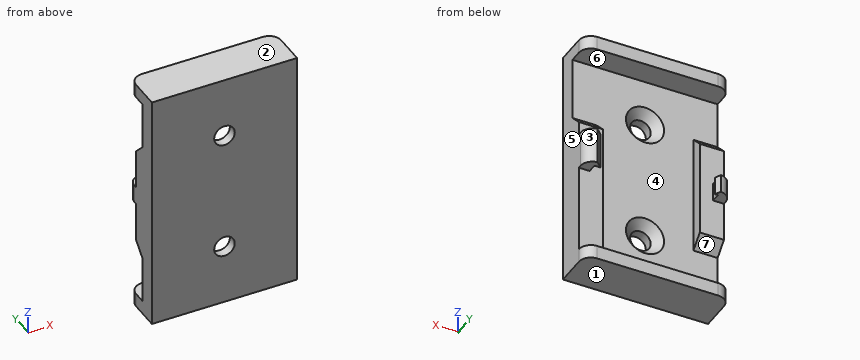
Autodesk Inventor part; units mm, degrees
ref_plane "YZ Plane" through (0, 0, 0) normal (1, 0, 0) x (0, 1, 0)
ref_plane "XZ Plane" through (0, 0, 0) normal (0, 1, 0) x (-1, 0, 0)
ref_plane "XY Plane" through (0, 0, 0) normal (0, 0, 1) x (1, 0, 0)
sketch "Skizze1" plane through (0, 0, 0) normal (0, 1, 0) x (-1, 0, 0)
  line L0 (0, 0) -> (24, 0)
  line L1 (24, 0) -> (24, -40)
  line L2 (24, -40) -> (0, -40)
  line L3 (0, -40) -> (0, 0)
  dimension "d0" = 40
  dimension "d1" = 24
extrude "Extrusion1" add sketch "Skizze1" along normal blind 3
sketch "Skizze2" plane through (0, 3, 0) normal (0, 1, 0) x (1, 0, 0)
  line L0 (-24, 40) -> (-24, 0)
  line L1 (0, 0) -> (0, 40)
  line L2 (-24, 0) -> (0, 0)
  line L3 (0, 0) -> (0, 2.25)
  line L4 (0, 2.25) -> (-24, 2.25)
  line L5 (-24, 2.25) -> (-24, 0)
  line L6 (0, 40) -> (-24, 40)
  line L7 (-24, 40) -> (0, 40)
  line L8 (0, 40) -> (0, 37.75)
  line L9 (0, 37.75) -> (-24, 37.75)
  line L10 (-24, 37.75) -> (-24, 40)
  dimension "d4" = 2.25
  dimension "d5" = 2.25
extrude "Extrusion2" add sketch "Skizze2" along normal blind 4 contours L6 L1 L9 L0 | L4 L1 L2 L0
sketch "Skizze4" plane through (0, 3, 0) normal (0, 1, 0) x (1, 0, 0)
  line L0 (0, 2.25) -> (-24, 2.25)
  line L1 (0, 2.25) -> (-1.8184, 2.25)
  line L2 (0, 37.75) -> (-1.8184, 37.75)
  line L3 (-24.0183, 2.25) -> (-21.7244, 2.25)
  line L4 (-24, 37.75) -> (-21.1801, 37.75)
  line L5 (0, 37.75) -> (-4, 37.75)
  line L6 (-4, 37.75) -> (-4, 12.75)
  line L7 (-4, 12.75) -> (0, 12.75)
  line L8 (0, 12.75) -> (0, 37.75)
  line L9 (-24, 37.75) -> (-24, 2.25)
  line L10 (-24, 10) -> (-20, 10)
  line L11 (-20, 10) -> (-20, 30)
  line L12 (-20, 30) -> (-24, 30)
  line L13 (-24, 30) -> (-24, 10)
  line L14 (-24, 0) -> (0, 0)
  dimension "d25" = 25
  dimension "d26" = 4
  dimension "d27" = 4
  dimension "d29" = 20
  dimension "d30" = 10
extrude "Extrusion4" add sketch "Skizze4" along normal blind 2
sketch "Skizze5" plane through (0, 5, 0) normal (0, 1, 0) x (1, 0, 0)
  line L0 (-24, 30) -> (-24, 10)
  line L1 (-24, 20) -> (0, 20)
  line L2 (0, 0) -> (0, 40)
  line L3 (-24, 18.5) -> (-22.2, 18.5)
  line L4 (-22.2, 18.5) -> (-22.2, 21.5)
  line L5 (-22.2, 21.5) -> (-24, 21.5)
  line L6 (-24, 21.5) -> (-24, 18.5)
  line L7 (0, 17) -> (-1.8, 17)
  line L8 (-1.8, 17) -> (-1.8, 23)
  line L9 (-1.8, 23) -> (0, 23)
  line L10 (0, 23) -> (0, 17)
  point P0 (-23.1, 18.5)
  point P1 (0, 23)
  dimension "d33" = 3
  dimension "d34" = 1.8
  dimension "d35" = 1.8
  dimension "d36" = 6
extrude "Extrusion5" add sketch "Skizze5" along normal blind 2.5
sketch "Skizze6" plane through (-1.8, 5, -23) normal (-1, 0, 0) x (0, 0, 1)
  line L0 (0, 0) -> (0, 2.5)
  line L1 (6, 0) -> (6, 2.5)
  line L2 (0, 2.5) -> (6, 2.5)
  line L3 (6, 2.5) -> (6, 1.5)
  line L4 (6, 1.5) -> (0, 1.5)
  line L5 (0, 1.5) -> (0, 2.5)
  point P0 (23, -5)
  point P1 (0, 1.5)
  dimension "d39" = 1
extrude "Extrusion6" add sketch "Skizze6" along normal blind 1
sketch "Skizze7" plane through (0, 5, -23) normal (0, 0, -1) x (-1, 0, 0)
  line L0 (2.8, 2.5) -> (2.8, 1.5)
  line L1 (2.8, 1.5) -> (1.8, 2.5)
  line L2 (0, 2.5) -> (2.8, 2.5)
  line L3 (1.8, 2.5) -> (2.8, 2.5)
  line L4 (2.8, 2.5) -> (2.8, 1.5)
  point P0 (0, -5)
  dimension "d42" = 1
  dimension "d43" = 1
extrude "Extrusion7" cut sketch "Skizze7" against normal blind 10
sketch "Skizze9" plane through (-22.2, 5, -18.5) normal (1, 0, 0) x (0, 0, -1)
  line L0 (0, 0) -> (0, 2.5)
  line L1 (3, 0) -> (3, 2.5)
  line L2 (0, 2.5) -> (3, 2.5)
  line L3 (3, 2.5) -> (3, 1.5)
  line L4 (3, 1.5) -> (0, 1.5)
  line L5 (0, 1.5) -> (0, 2.5)
  line L6 (3, 0) -> (0, 0)
  point P0 (-18.5, -5)
  point P1 (0, 1.5)
  dimension "d46" = 1.5
extrude "Extrusion8" add sketch "Skizze9" along normal blind 0.5 contours L0 L2 L1 L4
sketch "Skizze11" plane through (-22.2, 5, -21.5) normal (0, 0, -1) x (-1, 0, 0)
  line L0 (-0.5, 2.5) -> (-0.5, 1.5)
  line L1 (-0.5, 1.5) -> (0, 2.5)
  line L2 (1.8, 2.5) -> (-0.5, 2.5)
  line L3 (-0.5, 1.5) -> (-0.5, 2.5)
  line L4 (-0.5, 2.5) -> (0, 2.5)
  point P0 (-22.2, -5)
  dimension "d49" = 0.5
extrude "Extrusion9" cut sketch "Skizze11" against normal blind 10
chamfer "Fasen1" distance 2 angle 45 3 edges at (-22, 5, -30) (-22, 5, -10) (-2, 5, -12.75)
fillet "Rundung1" radius 2 6 edges at (0, 7.5, -20) (-24, 7.5, -20) (-24, 7, -1.125) (0, 7, -1.125) (-24, 7, -38.875) (0, 7, -38.875)
sketch "Skizze12" plane through (0, 3, 0) normal (0, 1, 0) x (1, 0, 0)
  line L0 (-24, 0) -> (0, 0)
  line L1 (-12, 0) -> (-12, 40)
  line L2 (0, 40) -> (-24, 40)
  circle A0 centre (-12, 10) radius 2
  circle A1 centre (-12, 30) radius 2
  line L3 (-24, 40) -> (-24, 0)
  line L4 (-24, 20) -> (0, 20) construction
  line L5 (0, 17) -> (0, 23)
  dimension "d56" = 4
  dimension "d57" = 4
  dimension "d58" = 20
hole "Bohrung1" at (-12, 3, -10) at (-12, 3, -30) direction (0, -1, 0) diameter 3.4 depth 8.8 tip angle 118 countersink diameter 6.3 countersink angle 90
properties part number "Halter_Treiber_LED"
For this review, take the finished solid that the model builds, in its own axes (mm). Face numbers are marked on the shaded views. A direction names the side the tool comes from. Round coordinates to 2 decimals unless told otherwise and drop trailing zeros. Write each loop counter-clockwise with the first axis right and the second up, starting at its lowest first coordinate (ties: lowest second). Pieces come first, ordered by that corner, then holes.
1) Insertion check: pin 1 Ø1.1 at (x, z) = (-12.5, -38.5) entering from +Y. The pin has a flat end and moves straight along its axis. Give the tip position at first contact, or say it passes through.
Answer below:
pin 1: stops at y = 7
2) Take a section at C-C on x = -18. Give the boundary of the cut face in (y, z), then the cut area to 3 significant figures.
Answer below:
outline: (0, -40) - (7, -40) - (7, -37.75) - (3, -37.75) - (3, -2.25) - (7, -2.25) - (7, 0) - (0, 0) - close
area: 138 mm2
3) Take a section at D-D on y = 0.75. Give the boundary of the cut face in (x, z).
Answer below:
outline: (-24, -40) - (0, -40) - (0, 0) - (-24, 0) - close; hole circle Ø3.4 at (-12, -30); hole circle Ø3.4 at (-12, -10)
4) Machinability: for the marked faces 5, 6 and 7, which of the approach directions +Z, -Z, +X, -X, +Y, -Y give a long, thin tool a straight path to every point of the face, cutting with its end or side? Answer none if there is none.
Answer below:
face 5: +Z, -Z, +X, +Y, -Y
face 6: +X, -X, +Y
face 7: -X, +Y
5) For line 1 along Z through (x, y) = (-12, 0.4); line 2 along X through (y, z) = (0.8, -10); line 3 along Z through (x, y) = (-8.25, 4.75), list the stretches that pass through material, from the lowest coordinate up.
Answer below:
line 1: z = -40 to -31.7, -28.3 to -11.7, -8.3 to 0
line 2: x = -24 to -13.7, -10.3 to 0
line 3: z = -40 to -37.75, -2.25 to 0
6) Take a section at A-A on x = -12. Give the boundary of the cut face in (y, z).
Answer below:
outline: (0, -40) - (7, -40) - (7, -37.75) - (3, -37.75) - (3, -33.15) - (1.55, -31.7) - (0, -31.7) - close; (0, -28.3) - (1.55, -28.3) - (3, -26.85) - (3, -13.15) - (1.55, -11.7) - (0, -11.7) - close; (0, -8.3) - (1.55, -8.3) - (3, -6.85) - (3, -2.25) - (7, -2.25) - (7, 0) - (0, 0) - close
7) Take a section at B-B on y = 4.5. Give the boundary of the cut face in (x, z).
Answer below:
outline: (-24, -40) - (0, -40) - (0, -14.25) - (-4, -14.25) - (-4, -37.75) - (-24, -37.75) - close; (-24, -28.5) - (-20, -28.5) - (-20, -11.5) - (-24, -11.5) - close; (-24, -2.25) - (0, -2.25) - (0, 0) - (-24, 0) - close
8) Mouldability with a two-part tool opening along Z and no side actions: class the marked faces 1, 2, 3 and 4 as +Z half, -Z half, draft (parallel to the pull), parting line (faces both ways), or undercut.
Answer below:
face 1: -Z half
face 2: +Z half
face 3: draft
face 4: undercut
